Source: CAD feature listing. Evaluate the final solid. Frame: model axes, mm. Give positions to 0.01 mm unless a question says otherwise; leave off trailing zeros. Write each loop counter-clockwise with the first axis right and the second up, starting at its lowest first coordinate (ties: lowest second). Pieces come first, ordered by that corner, then holes. Notation, with made-up numbers: M 87.5,17.5 L 133.5,17.5 A21 cw 133.5,43.5 Z; hole C -37,52 d7. An arc over 180 degrees is marked long. Answer as a JSON object with one key per item and string values. Group by question number.
```python
from build123d import *

# Parameters (mm, degrees)
SKETCH_1_R             = 3.25
SKETCH_1_R_2           = 22.5
SM_BASE_FLANGE_1_DEPTH = 1.5


# Sheet-metal steps are written as plain solids
with BuildPart() as part:
    # Sketch 1 → Базовая кромка1 (new body)
    with BuildSketch(Plane.XY):
        with BuildLine():
            Line((677.266802552, -1.5), (677.266802552, -16.5))
            Line((677.266802552, -16.5), (-322.733197448, -16.5))
            Line((-322.733197448, -16.5), (-322.733197448, 4.22618932))
            Line((-322.733197448, 4.22618932), (-322.733197448, 28.22618932))
            ThreePointArc((-322.733197448, 28.22618932), (-323.611877105, 30.347509663), (-325.733197448, 31.22618932))
            Line((-325.733197448, 31.22618932), (-349.733197448, 31.22618932))
            ThreePointArc((-349.733197448, 31.22618932), (-351.854517792, 30.347509663), (-352.733197448, 28.22618932))
            Line((-352.733197448, 28.22618932), (-352.733197448, 4.22618932))
            Line((-352.733197448, 4.22618932), (-352.733197448, -16.5))
            Line((-352.733197448, -16.5), (-452.733197448, -16.5))
            Line((-452.733197448, -16.5), (-452.733197448, 4.22618932))
            Line((-452.733197448, 4.22618932), (-452.733197448, 28.22618932))
            ThreePointArc((-452.733197448, 28.22618932), (-453.611877105, 30.347509663), (-455.733197448, 31.22618932))
            Line((-455.733197448, 31.22618932), (-479.733197448, 31.22618932))
            ThreePointArc((-479.733197448, 31.22618932), (-481.854517792, 30.347509663), (-482.733197448, 28.22618932))
            Line((-482.733197448, 28.22618932), (-482.733197448, 4.22618932))
            Line((-482.733197448, 4.22618932), (-482.733197448, -16.5))
            Line((-482.733197448, -16.5), (-727.412308586, -16.5))
            Line((-727.412308586, -16.5), (-727.412308586, 0))
            Line((-727.412308586, 0), (-665.607683437, 169.806812014))
            Line((-665.607683437, 169.806812014), (-628.27182662, 272.386235556))
            ThreePointArc((-628.27182662, 272.386235556), (-625.181995264, 277.685039029), (-620.432527225, 281.566653306))
            Line((-620.432527225, 281.566653306), (-403.291964068, 401.983925448))
            ThreePointArc((-403.291964068, 401.983925448), (-397.280386008, 403.986243464), (-390.951446304, 403.681496942))
            Line((-390.951446304, 403.681496942), (571.017994956, 175.466516041))
            ThreePointArc((571.017994956, 175.466516041), (574.328905861, 174.314751992), (577.338388414, 172.517057299))
            Line((577.338388414, 172.517057299), (643.325554365, 123.355108982))
            Line((643.325554365, 123.355108982), (787.266802552, 16.115585934))
            Line((787.266802552, 16.115585934), (787.266802552, -16.5))
            Line((787.266802552, -16.5), (757.266802552, -16.5))
            Line((757.266802552, -16.5), (757.266802552, -1.5))
            Line((757.266802552, -1.5), (677.266802552, -1.5))
        make_face()
        with Locations((-417.733197448, 133.22618932)):
            Circle(SKETCH_1_R, mode=Mode.SUBTRACT)
        with Locations((-417.733197448, 103.22618932)):
            Circle(SKETCH_1_R_2, mode=Mode.SUBTRACT)
        with Locations((-391.752435335, 118.22618932)):
            Circle(SKETCH_1_R, mode=Mode.SUBTRACT)
        with Locations((-391.752435335, 88.22618932)):
            Circle(SKETCH_1_R, mode=Mode.SUBTRACT)
        with Locations((-417.733197448, 73.22618932)):
            Circle(SKETCH_1_R, mode=Mode.SUBTRACT)
        with Locations((-443.713959562, 88.22618932)):
            Circle(SKETCH_1_R, mode=Mode.SUBTRACT)
        with Locations((-443.713959562, 118.22618932)):
            Circle(SKETCH_1_R, mode=Mode.SUBTRACT)
    extrude(amount=SM_BASE_FLANGE_1_DEPTH)


solid = part.part
```
(1) Pull-direction query (X, two-part tool) for faces 1 (the flat face through (-128, 150, 1.5)), 2 (the cylindrical face through (-396.95, 94.61, 0.74)), 3 (the flat face through (83.3, 291.17, 0.74)); classes: pulls with the +X half, pulls with the -X half, needs draft (parallel to the pull), parting line crosses it, or undercut.
(2) Section A-A, the plane y = 317. Return loops of the section in (x, z), plus the area to 3 significant figures.
(3) Section C-C, the plane z = 1.05. State how many separate pieces and enclosed holes the cut face has, plus the area to 3 significant figures.
(4) Contact query for a flat-ended pin moving along its axis: pin 1 Ø0.8 at (x, z) = (-466, 0.5) entering from -Y. Output: stop coordinate, or through.
(5) Ray query, L1, parallel to X at y = 89, z = 0.1; L2, parallel to X at y = 106, z = 0.75; L3, parallel to Y at x = -80, z = 0.35. Return the intervals inside material, ascending. Write a range as [from, to].
(6) Section B-B, the plane x = -125. Return loops of the section in (y, z), plus the area to 3 significant figures.
Reported:
{
 "1": {"face 1": "needs draft", "face 2": "undercut", "face 3": "pulls with the +X half"},
 "2": {"outline": "M -556.54,0 L -25.57,0 L -25.57,1.5 L -556.54,1.5 Z", "area": "796 mm2"},
 "3": {"separate pieces": "1", "enclosed holes": "7", "area": "413,000 mm2"},
 "4": {"pin 1": "stops at y = 31.23"},
 "5": {"L1": "x = [-695.02, -446.87], [-440.56, -435.16], [-400.3, -394.91], [-388.6, 689.44]", "L2": "x = [-688.83, -440.06], [-395.4, 666.62]", "L3": "y = [-16.5, 329.91]"},
 "6": {"outline": "M -16.5,0 L 340.59,0 L 340.59,1.5 L -16.5,1.5 Z", "area": "536 mm2"}
}
